CAD build for the part. Positions are in the model's coordinates, mm. A direction names the side the tool comes from. Round coordinates to 2 decimals unless told otherwise and drop trailing zeros. Order: outer loops, then holes, each group sorted by start corner. A loop starts at its lowest first (then second) coordinate and runs counter-clockwise, first axis right, second up. Notation, with made-up numbers: (47.5, -19) -> (69.5, -19) arc R19 ccw to (69.5, 5) -> close; hole circle Ø4 at (40, 25.25). An arc over 180 degrees is marked (long way). Return JSON: item names as keys, results as strings. Group by question number.
Q1. Cut at C-C (z = 2). Write the cut outline in (x, y).
Q2. Flat gauge pins, fed straight in: pin 1 (3 mm diameter, centred on x = 0, y = 0, fed in from -Z); pin 2 (3 mm diameter, centred on x = -1, y = -0.5, fed in from -Z); pin 3 (3 mm diameter, centred on x = 1, z = -1.5, fed in from -Y); pin 4 (2 mm diameter, centred on x = 1, z = -1.5, fed in from +Y). Where does each tip first touch, or does it go through?
Q3. Cut at D-D (z = 3). Write the cut outline in (x, y) (1 decimal), then the cut area to 3 significant figures.
Q4. Which spindle directions (+Z, -Z, +X, -X, +Y, -Y) get a long thin tool onto all of the face, cutting with end or side? Do faces 1 (the cylindrical face through (-2.84, -0.63, 2.88)), 2 (the flat face through (-2, -1, -3.96)), 3 (the cylindrical face through (-2.577, -0.572, 1.72)). Say none if no direction does.
Q5. Mould opens along Y. For faces 4 (the flat face through (-2, -1, 3.96)), 5 (the cylindrical face through (-2, 0, 0)), 6 (the cylindrical face through (0.74, 2.34, -1.35)) say: +Y half, -Y half, draft (parallel to the pull), parting line (faces both ways), or undercut.
Q6. Probe line 1 along X through (y, z) = (0, 0.5); line 2 along Z through (x, y) = (-0.5, -2.5); line 3 along X through (y, z) = (0, -3). List the from-to ranges inside material, lowest first.
from build123d import *


with BuildPart() as part:
    # Sketch3 → Revolve1 (revolve)
    with BuildSketch(Plane(origin=(0, 0, 0), x_dir=(0, 0, -1), z_dir=(1, 0, 0))):
        Polygon((-3.96, 2), (-3.96, 3.175), (-3.4848, 3.175), (-3.4848, 2.9075), (-2.2968, 2.9075), (-2.2968, 2.64), (-1.158946666, 2.64), (-1.158946666, 2.9075), (-0.220748794, 2.9075), (0.8712, 2.4552), (1.814742989, 2.4552), (1.814742989, 2.77375), (2.583790719, 2.4552), (3.527333708, 2.4552), (3.527333708, 2.705), (3.96, 2.4552), (3.96, 2), align=None)
    revolve(axis=Axis((0, 0, 3.96), (0, 0, -1)))


solid = part.part
Solution:
{
 "1": {"outline": "circle Ø5.28 at (0, 0); hole circle Ø4 at (0, 0)"},
 "2": {"pin 1": "passes through", "pin 2": "stops at z = -3.96", "pin 3": "stops at y = -2.77", "pin 4": "stops at y = 2.77"},
 "3": {"outline": "circle Ø5.8 at (0, 0); hole circle Ø4 at (0, 0)", "area": "14.0 mm²"},
 "4": {"face 1": "-Z", "face 2": "-Z, +X, -X, +Y, -Y", "face 3": "none"},
 "5": {"face 4": "draft", "face 5": "undercut", "face 6": "parting line"},
 "6": {"line 1": "x = -2.91 to -2, 2 to 2.91", "line 2": "z = -3.8 to -3.53, -2.36 to -1.81, -0.64 to 3.96", "line 3": "x = -2.46 to -2, 2 to 2.46"}
}
